Geometry: final body of the model. Coordinates: model frame, mm. Give positions to 0.01 mm unless a question says otherwise; leave off trailing zeros. Write each loop counter-clockwise with the first axis right and the second up, starting at its lowest first coordinate (ties: lowest second). Pieces come first, ordered by that corner, then holes. Notation, with made-up numbers: (72, 32.5) -> (121, 32.5) arc R31 ccw to (121, 69.5) -> close; hole circle Ø11 at (13.25, -25). An arc over 180 degrees is marked (long way). Answer in a Markdown table with one row per item. Add a question column.
from build123d import *

# Parameters (mm, degrees)
F1_DEPTH = 2.5


with BuildPart() as f1:
    # F0 (on Top) → F1 (new body)
    with BuildSketch(Plane.XY):
        with BuildLine():
            ThreePointArc((-4.432018362, -59.389646693), (-9.2830207067, -61.3989976553), (-11.2923716689, -66.25))
            Line((-11.2923716689, -66.25), (-6.307018362, -66.25))
            ThreePointArc((-6.307018362, -66.25), (-5.7578435767, -64.9241747853), (-4.432018362, -64.375))
            Line((-4.432018362, -64.375), (-4.432018362, -59.389646693))
        make_face()
        with BuildLine():
            ThreePointArc((-11.2923716689, -66.25), (-11.0075540706, -68.2062151314), (-10.1767505138, -70))
            Line((-10.1767505138, -70), (-3.300883806, -70))
            Line((-3.300883806, -70), (-5.5188745002, -67.7778641088))
            ThreePointArc((-5.5188745002, -67.7778641088), (-5.7590807574, -67.5745868785), (-5.961909132, -67.3340014907))
            ThreePointArc((-5.961909132, -67.3340014907), (-6.2186590917, -66.8188056813), (-6.307018362, -66.25))
            Line((-6.307018362, -66.25), (-11.2923716689, -66.25))
        make_face()
        with BuildLine():
            Line((-3.300883806, -70), (-10.1767505138, -70))
            ThreePointArc((-10.1767505138, -70), (-9.6316427271, -70.7253049011), (-8.9955877088, -71.3723317262))
            ThreePointArc((-8.9955877088, -71.3723317262), (-5.1719813551, -73.0703300701), (-1.073184401, -72.2318627466))
            Line((-1.073184401, -72.2318627466), (-3.300883806, -70))
        make_face()
        with BuildLine():
            Line((-5.5188745002, -67.7778641088), (-3.300883806, -70))
            Line((-3.300883806, -70), (-0.682018362, -70))
            Line((-0.682018362, -70), (-0.682018362, -67.3733334464))
            Line((-0.682018362, -67.3733334464), (-2.9275173343, -65.1310265161))
            ThreePointArc((-2.9275173343, -65.1310265161), (-2.6520514484, -65.6606420557), (-2.557018362, -66.25))
            ThreePointArc((-2.557018362, -66.25), (-3.5724342355, -67.9163553431), (-5.5188745002, -67.7778641088))
        make_face()
        with BuildLine():
            ThreePointArc((-0.682018362, -60.5052678482), (-2.4758032306, -59.6744642913), (-4.432018362, -59.389646693))
            Line((-4.432018362, -59.389646693), (-4.432018362, -64.375))
            ThreePointArc((-4.432018362, -64.375), (-3.8439266036, -64.4696143441), (-3.3151862223, -64.7439087107))
            ThreePointArc((-3.3151862223, -64.7439087107), (-3.1071365022, -64.9232321011), (-2.9275173343, -65.1310265161))
            Line((-2.9275173343, -65.1310265161), (-0.682018362, -67.3733334464))
            Line((-0.682018362, -67.3733334464), (-0.682018362, -60.5052678482))
        make_face()
        with BuildLine():
            Line((-0.682018362, -60.5052678482), (-0.682018362, -67.3733334464))
            Line((-0.682018362, -67.3733334464), (1.5522932658, -69.6044689353))
            ThreePointArc((1.5522932658, -69.6044689353), (2.2057124085, -67.9834871547), (2.428334945, -66.25))
            ThreePointArc((2.428334945, -66.25), (1.9563934061, -63.7494715403), (0.6055009602, -61.5929787873))
            Line((0.6055009602, -61.5929787873), (0.2178320688, -61.2058609786))
            ThreePointArc((0.2178320688, -61.2058609786), (-0.2175101465, -60.8368338287), (-0.682018362, -60.5052678482))
        make_face()
        with BuildLine():
            Line((-0.682018362, -70), (-3.300883806, -70))
            Line((-3.300883806, -70), (-1.073184401, -72.2318627466))
            ThreePointArc((-1.073184401, -72.2318627466), (0.4207532103, -71.0992324716), (1.5522932658, -69.6044689353))
            Line((1.5522932658, -69.6044689353), (-0.682018362, -67.3733334464))
            Line((-0.682018362, -67.3733334464), (-0.682018362, -70))
        make_face()
        with BuildLine():
            ThreePointArc((-1.073184401, -72.2318627466), (-5.1719813551, -73.0703300701), (-8.9955877088, -71.3723317262))
            Line((-8.9955877088, -71.3723317262), (5.8543275971, -86.25))
            Line((5.8543275971, -86.25), (8.692981638, -86.25))
            ThreePointArc((8.692981638, -86.25), (8.9153876284, -84.5154631906), (9.5682159488, -82.8931507817))
            Line((9.5682159488, -82.8931507817), (-1.073184401, -72.2318627466))
        make_face()
        with BuildLine():
            ThreePointArc((1.5522932658, -69.6044689353), (0.4207532103, -71.0992324716), (-1.073184401, -72.2318627466))
            Line((-1.073184401, -72.2318627466), (9.5682159488, -82.8931507817))
            ThreePointArc((9.5682159488, -82.8931507817), (10.7071629023, -81.3881005545), (12.2124662871, -80.249488211))
            Line((12.2124662871, -80.249488211), (1.5522932658, -69.6044689353))
        make_face()
        with BuildLine():
            ThreePointArc((2.428334945, -66.25), (2.2057124085, -67.9834871547), (1.5522932658, -69.6044689353))
            Line((1.5522932658, -69.6044689353), (12.2124662871, -80.249488211))
            ThreePointArc((12.2124662871, -80.249488211), (13.8341842954, -79.5972132324), (15.567981638, -79.375))
            Line((15.567981638, -79.375), (15.567981638, -76.5341898643))
            Line((15.567981638, -76.5341898643), (0.6055009602, -61.5929787873))
            ThreePointArc((0.6055009602, -61.5929787873), (1.9563934061, -63.7494715403), (2.428334945, -66.25))
        make_face()
        with BuildLine():
            ThreePointArc((15.567981638, -79.375), (13.8341842954, -79.5972132324), (12.2124662871, -80.249488211))
            Line((12.2124662871, -80.249488211), (15.567981638, -83.6002335993))
            Line((15.567981638, -83.6002335993), (15.567981638, -79.375))
        make_face()
        with BuildLine():
            ThreePointArc((12.2124662871, -80.249488211), (10.7071629023, -81.3881005545), (9.5682159488, -82.8931507817))
            Line((9.5682159488, -82.8931507817), (12.9188032632, -86.25))
            Line((12.9188032632, -86.25), (13.692981638, -86.25))
            ThreePointArc((13.692981638, -86.25), (14.2421564233, -84.9241747853), (15.567981638, -84.375))
            Line((15.567981638, -84.375), (15.567981638, -83.6002335993))
            Line((15.567981638, -83.6002335993), (12.2124662871, -80.249488211))
        make_face()
        with BuildLine():
            Line((12.9188032632, -86.25), (9.5682159488, -82.8931507817))
            ThreePointArc((9.5682159488, -82.8931507817), (8.9153876284, -84.5154631906), (8.692981638, -86.25))
            Line((8.692981638, -86.25), (12.9188032632, -86.25))
        make_face()
        with BuildLine():
            Line((8.692981638, -86.25), (5.8543275971, -86.25))
            Line((5.8543275971, -86.25), (9.5973323053, -90))
            Line((9.5973323053, -90), (9.8057663522, -90))
            ThreePointArc((9.8057663522, -90), (8.9770463823, -88.2058112013), (8.692981638, -86.25))
        make_face()
        with BuildLine():
            Line((15.567981638, -76.5341898643), (15.567981638, -79.375))
            ThreePointArc((15.567981638, -79.375), (17.5237928393, -79.6590647443), (19.317981638, -80.4877847142))
            Line((19.317981638, -80.4877847142), (19.317981638, -80.2788591303))
            Line((19.317981638, -80.2788591303), (15.567981638, -76.5341898643))
        make_face()
        with BuildLine():
            Line((13.692981638, -86.25), (12.9188032632, -86.25))
            Line((12.9188032632, -86.25), (14.2409192426, -87.5745868785))
            ThreePointArc((14.2409192426, -87.5745868785), (13.8353727682, -86.9667227527), (13.692981638, -86.25))
        make_face()
        with BuildLine():
            Line((16.8928634978, -84.9232321011), (15.567981638, -83.6002335993))
            Line((15.567981638, -83.6002335993), (15.567981638, -84.375))
            ThreePointArc((15.567981638, -84.375), (16.2848969711, -84.5174708068), (16.8928634978, -84.9232321011))
        make_face()
        with BuildLine():
            Line((12.9188032632, -86.25), (8.692981638, -86.25))
            ThreePointArc((8.692981638, -86.25), (8.9770463823, -88.2058112013), (9.8057663522, -90))
            Line((9.8057663522, -90), (19.317981638, -90))
            Line((19.317981638, -90), (19.317981638, -80.4877847142))
            ThreePointArc((19.317981638, -80.4877847142), (17.5237928393, -79.6590647443), (15.567981638, -79.375))
            Line((15.567981638, -79.375), (15.567981638, -83.6002335993))
            Line((15.567981638, -83.6002335993), (16.8928634978, -84.9232321011))
            ThreePointArc((16.8928634978, -84.9232321011), (17.3000004727, -85.5318525524), (17.442981638, -86.25))
            ThreePointArc((17.442981638, -86.25), (16.2847043907, -87.9826088698), (14.2409192426, -87.5745868785))
            Line((14.2409192426, -87.5745868785), (12.9188032632, -86.25))
        make_face()
        with BuildLine():
            Line((19.317981638, -90), (9.8057663522, -90))
            ThreePointArc((9.8057663522, -90), (10.2251877733, -90.5766821837), (10.7020861881, -91.1068185544))
            ThreePointArc((10.7020861881, -91.1068185544), (18.1959650647, -92.6028991893), (22.442981638, -86.25))
            ThreePointArc((22.442981638, -86.25), (21.9187173646, -83.6167926912), (20.4258817889, -81.385184369))
            ThreePointArc((20.4258817889, -81.385184369), (19.8952576619, -80.9076870915), (19.317981638, -80.4877847142))
            Line((19.317981638, -80.4877847142), (19.317981638, -90))
        make_face()
    extrude(amount=F1_DEPTH)


solid = f1.part
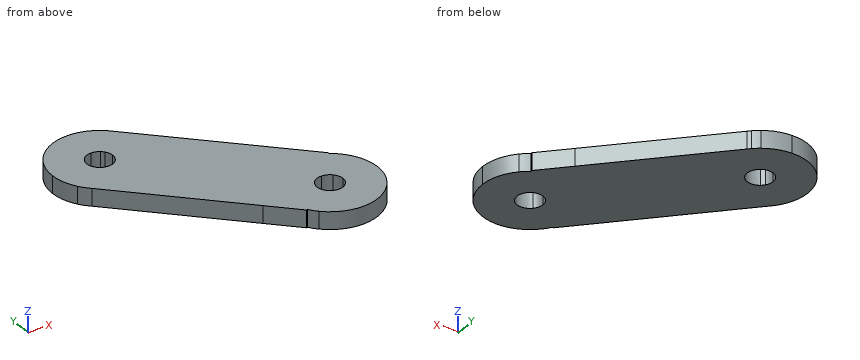
Q1. Section A-A on z = 0.9. Count the separate pieces of the cut face and the enclosed holes in it, and give its area (3 significant figures).
Q2. Line query: probe 1 along Y at (x, z) = (15.5, 1.45); probe 2 along X at (y, z) = (-65, 1); probe 3 along X at (y, z) = (-66.5, 1.5). Output: solid intervals per line, ascending. Write a range as from..to.
Q3. Contact query for a flat-ended pin moving along its axis: pin 1 Ø1 at (x, y) = (13.5, -81) entering from -Z. Output: stop coordinate, or through.
Q4. Section C-C on y = -78. Return loops of the section in (x, z).
Q5. Section D-D on y = -83. Return loops of the section in (x, z), and give its area (3 significant figures).
Q6. Section B-B on x = -5. Return loops of the section in (y, z), and give its area (3 significant figures).
Checks:
| question | item | result |
|---|---|---|
| 1 | separate pieces | 1 |
| 1 | enclosed holes | 2 |
| 1 | area | 514 mm^2 |
| 2 | probe 1 | -93.12..-88.12, -84.38..-76.47 |
| 2 | probe 2 | -11.18..-5.83, -3.03..4.02 |
| 2 | probe 3 | -11.29..-6.29, -2.57..5.52 |
| 3 | pin 1 | z = 0 |
| 4 | outline | (-2.38, 0) -> (17.04, 0) -> (17.04, 2.5) -> (-2.38, 2.5) -> close |
| 5 | outline | (2.61, 0) -> (21.63, 0) -> (21.63, 2.5) -> (2.61, 2.5) -> close |
| 5 | area | 47.5 mm^2 |
| 6 | outline | (-75.38, 0) -> (-68.04, 0) -> (-68.04, 2.5) -> (-75.38, 2.5) -> close; (-64.46, 0) -> (-59.41, 0) -> (-59.41, 2.5) -> (-64.46, 2.5) -> close |
| 6 | area | 31.0 mm^2 |
